Can you work these out from the model? Positions are in its coordinate system, mm. A direction names the side the tool comes from. Round coordinates to 2 decimals unless told otherwise and drop trailing zeros. Write item = value, one per line.
from build123d import *

# Parameters (mm, degrees)
SKETCH2_R            = 15
BOSS_EXTRUDE1_DEPTH  = 5
SKETCH3_R            = 10
CUT_EXTRUDE1_DEPTH   = 2
M3_CLEARANCE_HOLE1_D = 3.6
FILLET1_R            = 10


with BuildPart() as part:
    # Sketch2 → Boss-Extrude1 (new body)
    with BuildSketch(Plane(origin=(0, 0, 0), x_dir=(1, 0, 0), z_dir=(0, 1, 0))):
        with Locations(Location((0, 0, 0), (0, 0, 270))):
            Circle(SKETCH2_R)
    extrude(amount=BOSS_EXTRUDE1_DEPTH)

    # Sketch3 → Cut-Extrude1 (cut)
    with BuildSketch(Plane.XZ):
        with Locations(Location((0, 0, 0), (0, 0, 270))):
            Circle(SKETCH3_R)
    extrude(amount=-CUT_EXTRUDE1_DEPTH, mode=Mode.SUBTRACT)

    # M3 Clearance Hole1 (through all)
    with Locations(Plane(origin=(0, 5, 0), x_dir=(1, 0, 0), z_dir=(0, 1, 0))):
        with Locations((0, 0)):
            Hole(M3_CLEARANCE_HOLE1_D / 2)

    # Fillet1
    # the kernel refuses this fillet: 10 mm, written as the material it takes off along each edge
    with BuildSketch(Plane(origin=(0, 5, 0), x_dir=(0, 0, 1), z_dir=(-1, 0, 0))) as fillet1_piece_1:
        with BuildLine():
            CenterArc((6.339745962, -10), FILLET1_R, 30, 60)
            Line((6.339745962, 0), (6.339745962, 0.2))
            Line((6.339745962, 0.2), (15, 0.2))
            Line((15, 0.2), (15.2, 0))
            ThreePointArc((15.2, 0), (15.2, -2.5), (15.173205081, -4.9))
            Line((15.173205081, -4.9), (15, -5))
        make_face()
    revolve(axis=Axis((0, 5, 0), (0, 1, 0)), mode=Mode.SUBTRACT)


solid = part.part
(1) Will these pins go through, and if not, where does the flat tip stop? P1, Ø10, axis at x = -2.5, z = 2.5, coming from the -Y side; P2, Ø1.5, axis at y = 4.5, z = -5.5, coming from the +X side; P3, Ø2, axis at y = 3.5, z = -1.5, coming from the -X side.
Computed:
P1 = 2
P2 = 9.79
P3 = -12.87
(2) On a 3-axis mill with a long thin cutter (end or side, diameter ignored), from which of +Z, -Z, +X, -X, +Y, -Y can I reach the whole of each face in a straight line? I mean faces 4 (the face through (-10, 0, 3)), 5 (the face through (0, 2, -2)). Say none if no direction works.
Computed:
face_4 = +Z, -Z, +X, -X, -Y
face_5 = -Y
(3) If I drill on line 1 (Z direction, x = -4.5, y = 0.6); line 2 (Y direction, x = 6, z = -1.5); line 3 (Z direction, x = 0, y = 2.6), over which ranges is the centre line in solid material (lowest first)? Write a range as from..to.
Computed:
line_1 = -13.92..-8.93, 8.93..13.92
line_2 = 2..5
line_3 = -12.84..-1.8, 1.8..12.84
(4) Thinking about a two-plate mould opening in X: for faces 1 (the face through (-9.76, 0.99, 2.17)), 2 (the face through (-1.3, 5, -1.5)), 3 (the face through (-1.717, 3.479, -0.541)), which applies, +X half, -X half, draft (parallel to the pull), parting line (faces both ways), or undercut?
Computed:
face_1 = undercut
face_2 = draft
face_3 = undercut
